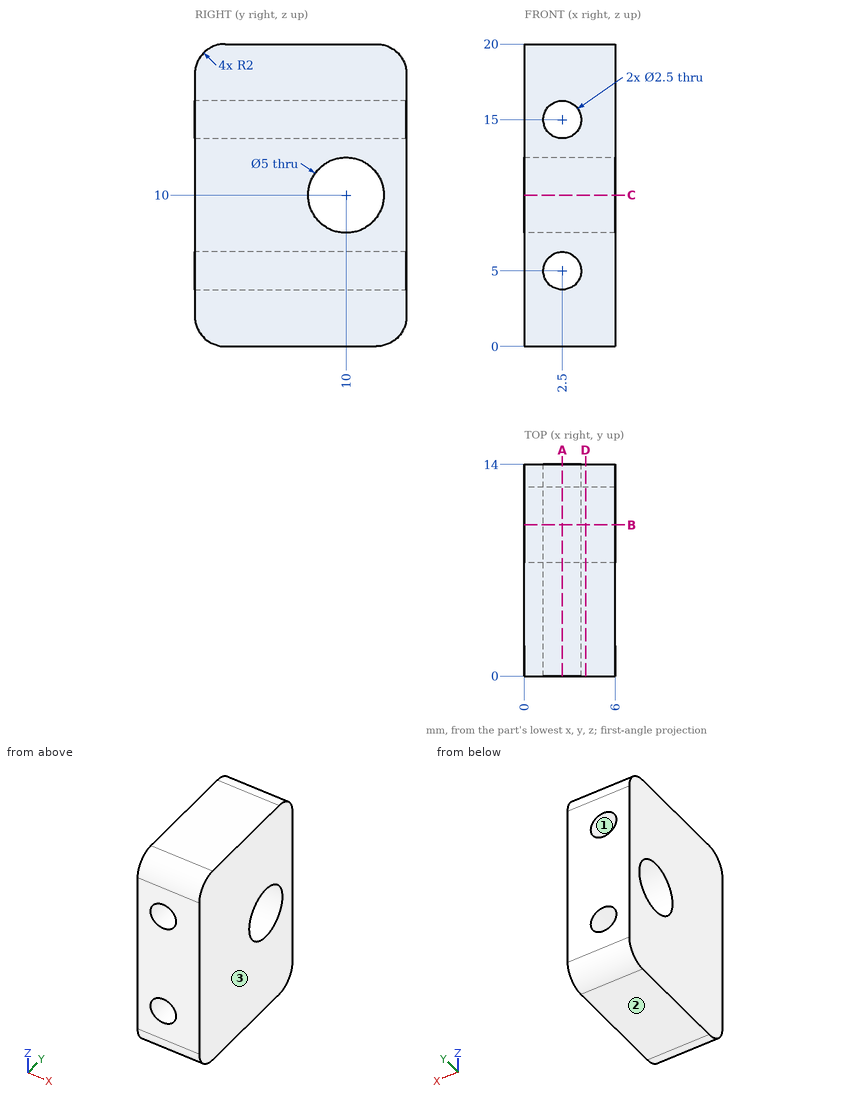
Job drawing, mm, ordinate dimensions from the low corner. One solid piece. Round coordinates to 2 decimals unless told otherwise and drop trailing zeros. Loops run counter-clockwise (first coordinate to the right, second up) from the corner with the lowest first, then second, coordinate; pieces in that order, holes last.
Item 1: Mould opens along Z. For the marked faces 1, 2 and 3 say: +Z half, -Z half, draft (parallel to the pull), parting line (faces both ways), or undercut.
Item 2: Drop a flat-ended pin along its axis: P1, Ø2, axis at x = 2.5, z = 15, coming from the +Y side. Give the stop position or say it passes through.
Item 3: Cut at C-C, the plane z = 10. Give the cut face in (x, y), then the cut area to 3 significant figures.
Item 4: Drill centre lines: line 1 (Y direction, x = 4.45, z = 10); line 2 (X direction, y = 7.5, z = 15); line 3 (Z direction, x = 2, y = 11.5). Where is each one in solid material? Low to high.
Item 5: Cut at D-D, the plane x = 4.05. Give the cut face in (y, z), then the cut area to 3 significant figures.
Item 6: Cut at B-B, the plane y = 10. Give the cut face in (x, z), then the cut area to 3 significant figures.
Item 7: Cut at A-A, the plane x = 2.5. Give the cut face in (y, z).
A:
1. face 1: undercut
1. face 2: -Z half
1. face 3: draft
2. P1: passes through
3. outline: (0, 0) - (6, 0) - (6, 7.5) - (0, 7.5) - close; (0, 12.5) - (6, 12.5) - (6, 14) - (0, 14) - close
3. area: 54.0 mm2
4. line 1: y = 0 to 7.5, 12.5 to 14
4. line 2: x = 0 to 1.25, 3.75 to 6
4. line 3: z = 0 to 3.85, 6.15 to 8, 12 to 13.85, 16.15 to 20
5. outline: (0, 2) arc R2 ccw to (2, 0) - (12, 0) arc R2 ccw to (14, 2) - (14, 18) arc R2 ccw to (12, 20) - (2, 20) arc R2 ccw to (0, 18) - close; hole circle Ø5 at (10, 10)
5. area: 257 mm2
6. outline: (0, 0) - (6, 0) - (6, 7.5) - (0, 7.5) - close; (0, 12.5) - (6, 12.5) - (6, 20) - (0, 20) - close; hole circle Ø2.5 at (2.5, 5); hole circle Ø2.5 at (2.5, 15)
6. area: 80.2 mm2
7. outline: (0, 2) arc R2 ccw to (2, 0) - (12, 0) arc R2 ccw to (14, 2) - (14, 3.75) - (0, 3.75) - close; (0, 6.25) - (14, 6.25) - (14, 13.75) - (0, 13.75) - close; (0, 16.25) - (14, 16.25) - (14, 18) arc R2 ccw to (12, 20) - (2, 20) arc R2 ccw to (0, 18) - close; hole circle Ø5 at (10, 10)
